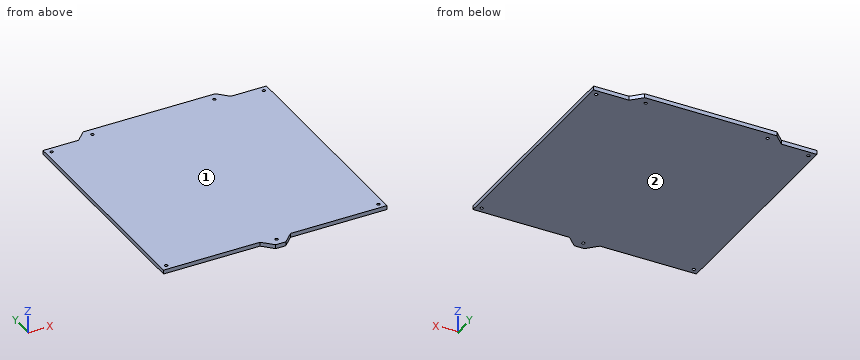
```python
from build123d import *

# Parameters (mm, degrees)
F0_R     = 1.5
F1_DEPTH = 4


with BuildPart() as f1:
    # F0 (on Top) → F1 (new body)
    with BuildSketch(Plane.XY):
        Polygon((-75, 110), (-110, 110), (-110, -110), (-15, -110), (-5, -120), (0, -120), (5, -120), (15, -110), (110, -110), (110, 110), (75, 110), (65, 120), (0, 120), (-65, 120), align=None)
        with Locations((-104.5, -104.5)):
            Circle(F0_R, mode=Mode.SUBTRACT)
        with Locations((0, -112.5)):
            Circle(F0_R, mode=Mode.SUBTRACT)
        with Locations((104.5, -104.5)):
            Circle(F0_R, mode=Mode.SUBTRACT)
        with Locations((-104.5, 104.5)):
            Circle(F0_R, mode=Mode.SUBTRACT)
        with Locations((-60, 112.5)):
            Circle(F0_R, mode=Mode.SUBTRACT)
        with Locations((60, 112.5)):
            Circle(F0_R, mode=Mode.SUBTRACT)
        with Locations((104.5, 104.5)):
            Circle(F0_R, mode=Mode.SUBTRACT)
    extrude(amount=F1_DEPTH)


solid = f1.part
```
Source: CAD feature listing. Evaluate the final solid. Frame: model axes, mm. Face numbers are marked on the shaded views. Round coordinates to 2 decimals unless told otherwise and drop trailing zeros. Order: outer loops, then holes, each group sorted by start corner. A loop starts at its lowest first (then second) coordinate and runs counter-clockwise, first axis right, second up. Notation, with made-up numbers: (21, -37.5) -> (72, -37.5) arc R28 ccw to (72, -7.5) -> close; hole circle Ø2 at (8.5, 27). An arc over 180 degrees is marked (long way). One line per item, written item: value. Start each with the question number.
Q1. Draft query along Z for the marked faces 1 and 2. Return one class per face: pulls with the +Z half, pulls with the -Z half, needs draft (parallel to the pull), parting line crosses it, or undercut.
Q2. Section query B-B (x = -53). Return the cut outline in (y, z).
Q3. Section query C-C (x = -9). Return the cut outline in (y, z), plus the area to 3 significant figures.
Q4. Pin query (flat end, axial travel): pin 1 (1 mm diameter, centred on x = 35.5, z = 2, fed in from -Y). Return the tip coordinate at first contact, or that it passes through.
Q5. Material intervals for probe 1 along X at (y, z) = (104.5, 1.95); probe 2 along X at (y, z) = (112.5, 2.2), sorted ascending.
Q6. Section query A-A (z = 1.6). Return the cut outline in (x, y).
Findings below:
1. face 1: pulls with the +Z half
1. face 2: pulls with the -Z half
2. outline: (-110, 0) -> (120, 0) -> (120, 4) -> (-110, 4) -> close
3. outline: (-116, 0) -> (120, 0) -> (120, 4) -> (-116, 4) -> close
3. area: 944 mm²
4. pin 1: y = -110
5. probe 1: -110 to -106, -103 to 103, 106 to 110
5. probe 2: -72.5 to -61.5, -58.5 to 58.5, 61.5 to 72.5
6. outline: (-110, -110) -> (-15, -110) -> (-5, -120) -> (5, -120) -> (15, -110) -> (110, -110) -> (110, 110) -> (75, 110) -> (65, 120) -> (-65, 120) -> (-75, 110) -> (-110, 110) -> close; hole circle Ø3 at (-104.5, -104.5); hole circle Ø3 at (-104.5, 104.5); hole circle Ø3 at (-60, 112.5); hole circle Ø3 at (0, -112.5); hole circle Ø3 at (60, 112.5); hole circle Ø3 at (104.5, -104.5); hole circle Ø3 at (104.5, 104.5)
